```python
from build123d import *

# Parameters (mm, degrees)
SKETCH_6_W           = 28.99281841
SKETCH_6_H           = 28.951324053
EXTRUDE_2_DEPTH      = 10
SKETCH_8_W           = 76
SKETCH_8_H           = 88
EXTRUDE_3_DEPTH      = 4
SKETCH_4_R           = 1.55
CUT_EXTRUDE_2_DEPTH  = 15
SKETCH_5_R           = 1.55
CUT_EXTRUDE_3_DEPTH  = 15
SKETCH_10_W          = 4.022554567
SKETCH_10_H          = 29.702617941
EXTRUDE_9_DEPTH      = 38
SKETCH_11_W          = 4.010171553
SKETCH_11_H          = 29.702617961
EXTRUDE_10_DEPTH     = 38
SKETCH_14_W          = 5
SKETCH_14_H          = 88
EXTRUDE_14_DEPTH     = 50
SKETCH_15_W          = 5
SKETCH_15_H          = 88
EXTRUDE_15_DEPTH     = 50
SKETCH_21_R          = 1.4
CUT_EXTRUDE_8_DEPTH  = 8
CUT_EXTRUDE_9_DEPTH  = 80
CUT_EXTRUDE_11_DEPTH = 80
FILLET_1_R           = 5
FILLET_2_R           = 5
SKETCH_24_W          = 28.984243656
SKETCH_24_H          = 0.299988544
EXTRUDE_16_DEPTH     = 10
SKETCH_25_W          = 37.016969776
SKETCH_25_H          = 2
EXTRUDE_18_DEPTH     = 10
FILLET_7_R           = 2
FILLET_8_R           = 3
FILLET_9_R           = 3
FILLET_10_R          = 3
SKETCH_19_R          = 3.1
CUT_EXTRUDE_12_DEPTH = 3
SKETCH_27_R          = 1.5
CUT_EXTRUDE_13_DEPTH = 10
SKETCH_28_R          = 1.6
CUT_EXTRUDE_15_DEPTH = 15


with BuildPart() as part:
    # 草图6 → 凸台-拉伸2 (new body)
    with BuildSketch(Plane.XZ.offset(14.4)):
        with Locations((0.000972868, 14.775650571)):
            Rectangle(SKETCH_6_W, SKETCH_6_H)
    extrude(amount=EXTRUDE_2_DEPTH)

    # 草图8 → 凸台-拉伸3 (add)
    with BuildSketch(Plane.XZ.offset(24.4)):
        with Locations((1e-09, -13.999999049)):
            Rectangle(SKETCH_8_W, SKETCH_8_H)
    extrude(amount=EXTRUDE_3_DEPTH)

    # 草图4 → 切除-拉伸2 (cut)
    with BuildSketch(Plane.XZ.offset(14.4)):
        with Locations(Location((-10, 2.1, 0), (0, 0, 270))):
            Circle(SKETCH_4_R)
        with Locations(Location((10, 2.1, 0), (0, 0, 270))):
            Circle(SKETCH_4_R)
    extrude(amount=CUT_EXTRUDE_2_DEPTH, mode=Mode.SUBTRACT)

    # 草图5 → 切除-拉伸3 (cut)
    with BuildSketch(Plane.XZ.offset(14.4)):
        with Locations(Location((0, 25.8, 0), (0, 0, 270))):
            Circle(SKETCH_5_R)
    extrude(amount=CUT_EXTRUDE_3_DEPTH, mode=Mode.SUBTRACT)

    # 草图10 → 凸台-拉伸9 (add)
    with BuildSketch(Plane(origin=(0, -24.4, 0), x_dir=(1, 0, 0), z_dir=(0, 1, 0))):
        with Locations((16.503397967, -14.851308971)):
            Rectangle(SKETCH_10_W, SKETCH_10_H)
    extrude(amount=EXTRUDE_9_DEPTH)

    # 草图11 → 凸台-拉伸10 (add)
    with BuildSketch(Plane(origin=(0, -24.4, 0), x_dir=(1, 0, 0), z_dir=(0, 1, 0))):
        with Locations((-16.497208749, -14.851308981)):
            Rectangle(SKETCH_11_W, SKETCH_11_H)
    extrude(amount=EXTRUDE_10_DEPTH)

    # 草图14 → 凸台-拉伸14 (add)
    with BuildSketch(Plane(origin=(0, -24.4, 0), x_dir=(1, 0, 0), z_dir=(0, 1, 0))):
        with Locations((-35.499999999, 13.999999049)):
            Rectangle(SKETCH_14_W, SKETCH_14_H)
    extrude(amount=EXTRUDE_14_DEPTH)

    # 草图15 → 凸台-拉伸15 (add)
    with BuildSketch(Plane(origin=(0, -24.4, 0), x_dir=(1, 0, 0), z_dir=(0, 1, 0))):
        with Locations((35.500000001, 13.999999049)):
            Rectangle(SKETCH_15_W, SKETCH_15_H)
    extrude(amount=EXTRUDE_15_DEPTH)

    # 草图21 → 切除-拉伸8 (cut)
    with BuildSketch(Plane(origin=(0, 25.6, 0), x_dir=(1, 0, 0), z_dir=(0, 1, 0))):
        with Locations(Location((-35.499999999, 52.999999049, 0), (0, 0, 270))):
            Circle(SKETCH_21_R)
        with Locations(Location((-35.499999999, -25.000000951, 0), (0, 0, 270))):
            Circle(SKETCH_21_R)
        with Locations(Location((35.500000001, 52.999999049, 0), (0, 0, 270))):
            Circle(SKETCH_21_R)
        with Locations(Location((35.500000001, -25.000000951, 0), (0, 0, 270))):
            Circle(SKETCH_21_R)
    extrude(amount=-CUT_EXTRUDE_8_DEPTH, mode=Mode.SUBTRACT)

    # 草图22 → 切除-拉伸9 (cut)
    with BuildSketch(Plane.ZY.offset(37.999999999)):
        with BuildLine():
            Line((-37.999999049, 10), (-17.999999049, 10))
            ThreePointArc((-17.999999049, 10), (-7.999999049, 0), (-17.999999049, -10))
            Line((-17.999999049, -10), (-37.999999049, -10))
            ThreePointArc((-37.999999049, -10), (-47.999999049, 0), (-37.999999049, 10))
        make_face()
    extrude(amount=-CUT_EXTRUDE_9_DEPTH, mode=Mode.SUBTRACT)

    # 草图23 → 切除-拉伸11 (cut)
    with BuildSketch(Plane(origin=(0, -24.4, 0), x_dir=(1, 0, 0), z_dir=(0, 1, 0))):
        with BuildLine():
            Line((10, 37.999999049), (10, 17.999999049))
            ThreePointArc((10, 17.999999049), (0, 7.999999049), (-10, 17.999999049))
            Line((-10, 17.999999049), (-10, 37.999999049))
            ThreePointArc((-10, 37.999999049), (0, 47.999999049), (10, 37.999999049))
        make_face()
    extrude(amount=-CUT_EXTRUDE_11_DEPTH, mode=Mode.SUBTRACT)

    # 圆角1
    fillet_1_edges = [part.edges().sort_by_distance(p)[0] for p in [
        (-32.999999999, -24.4, -13.999999049),
    ]]
    fillet(fillet_1_edges, radius=FILLET_1_R)

    # 圆角2
    fillet_2_edges = [part.edges().sort_by_distance(p)[0] for p in [
        (33.000000001, -24.4, -13.999999049),
    ]]
    fillet(fillet_2_edges, radius=FILLET_2_R)

    # 草图24 → 凸台-拉伸16 (add)
    with BuildSketch(Plane(origin=(0, -24.4, 0), x_dir=(1, 0, 0), z_dir=(0, 1, 0))):
        with Locations((-1.144e-06, -0.149994272)):
            Rectangle(SKETCH_24_W, SKETCH_24_H)
    extrude(amount=EXTRUDE_16_DEPTH)

    # 草图25 → 凸台-拉伸18 (add)
    with BuildSketch(Plane(origin=(0, -24.4, 0), x_dir=(1, 0, 0), z_dir=(0, 1, 0))):
        with Locations((0.006190363, 1)):
            Rectangle(SKETCH_25_W, SKETCH_25_H)
    extrude(amount=EXTRUDE_18_DEPTH)

    # 圆角7
    fillet_7_edges = [part.edges().sort_by_distance(p)[0] for p in [
        (0.006190363, -14.4, -2),
    ]]
    fillet(fillet_7_edges, radius=FILLET_7_R)

    # 圆角8
    fillet_8_edges = [part.edges().sort_by_distance(p)[0] for p in [
        (18.514675251, -24.4, 13.85130897),
    ]]
    fillet(fillet_8_edges, radius=FILLET_8_R)

    # 圆角9
    fillet_9_edges = [part.edges().sort_by_distance(p)[0] for p in [
        (1.506190363, -24.4, -2),
    ]]
    fillet(fillet_9_edges, radius=FILLET_9_R)

    # 圆角10
    fillet_10_edges = [part.edges().sort_by_distance(p)[0] for p in [
        (-18.502294525, -24.4, 12.35130898),
    ]]
    fillet(fillet_10_edges, radius=FILLET_10_R)

    # 草图19 → 切除-拉伸12 (cut)
    with BuildSketch(Plane.XZ.offset(28.4)):
        with Locations(Location((0, 25.8, 0), (0, 0, 270))):
            Circle(SKETCH_19_R)
        with Locations(Location((-10, 2.1, 0), (0, 0, 270))):
            Circle(SKETCH_19_R)
        with Locations(Location((10, 2.1, 0), (0, 0, 270))):
            Circle(SKETCH_19_R)
    extrude(amount=-CUT_EXTRUDE_12_DEPTH, mode=Mode.SUBTRACT)

    # 草图27 → 切除-拉伸13 (cut)
    with BuildSketch(Plane(origin=(0, 25.6, 0), x_dir=(1, 0, 0), z_dir=(0, 1, 0))):
        with Locations(Location((35.500000001, 52.999999049, 0), (0, 0, 270))):
            Circle(SKETCH_27_R)
        with Locations(Location((-35.499999999, 52.999999049, 0), (0, 0, 270))):
            Circle(SKETCH_27_R)
        with Locations(Location((-35.499999999, -25.000000951, 0), (0, 0, 270))):
            Circle(SKETCH_27_R)
        with Locations(Location((35.500000001, -25.000000951, 0), (0, 0, 270))):
            Circle(SKETCH_27_R)
    extrude(amount=-CUT_EXTRUDE_13_DEPTH, mode=Mode.SUBTRACT)

    # 草图28 → 切除-拉伸15 (cut)
    with BuildSketch(Plane.XZ.offset(28.4)):
        with Locations(Location((-10, 2.1, 0), (0, 0, 270))):
            Circle(SKETCH_28_R)
        with Locations(Location((10, 2.1, 0), (0, 0, 270))):
            Circle(SKETCH_28_R)
        with Locations(Location((0, 25.8, 0), (0, 0, 270))):
            Circle(SKETCH_28_R)
    extrude(amount=-CUT_EXTRUDE_15_DEPTH, mode=Mode.SUBTRACT)


solid = part.part
```
Input: part model. Units: mm. Frame: model coordinates. A direction names the side the tool comes from. Coordinates: 2 decimals unless noted, no trailing zeros. Loops run counter-clockwise (first coordinate to the right, second up) from the corner with the lowest first, then second, coordinate; pieces in that order, holes last. Notation, with made-up numbers: M 5.5,10 L 39.5,10 A16 ccw 39.5,37 Z; hole C -28.75,-16 d1. An arc over 180 degrees is marked long. Use a Markdown table: item, result. Add a question column.
1) Pin query (flat end, axial travel): P1, Ø5, axis at x = -3.5, z = -42.5, coming from the -Y side; P2, Ø4, axis at x = -10, z = 2.1, coming from the +Y side; P3, Ø6, axis at x = -11.5, y = -13.5, coming from the -Z side; P4, Ø2, axis at x = -17, z = 19.5, coming from the +Y side. Return the tip coordinate at first contact, or that it passes through.
2) Section D-D, the plane z = 2.1. Give the number of separate pieces and of enclosed holes in the cut face, plus the area to 3 significant figures.
3) Set-up query: faces 4 (the flat face through (35, -10, -28)), 5 (the flat face through (16, -6, 29.703)), 6 (the cylindrical face through (0.27, -15, -1.43)), 7 (the flat face through (33, 3, -4)), 8 (the cylindrical face through (0.931, -26.921, 22.843)). Return all of +Z, -Z, +X, -X, +Y, -Y with unobstructed straight access to the full face (end or side cutting, diameter ignored); none if empty.
4) Section C-C, the plane x = 0. Return the cut outline in (y, z).
5) Draft query along Y for faces 1 (the cylindrical face through (35, 0, -48)), 2 (the cylindrical face through (0, -26, -8)), 3 (the cylindrical face through (31.5, -22.97, -14.62)). Return one class per face: +Y half, -Y half, draft (parallel to the pull), parting line (faces both ways), or undercut.
6) Section A-A, the plane x = -35.5. Return the cut outline in (y, z), plus the area to 3 significant figures.
7) Section B-B, the plane z = -19.5. Return the cut outline in (x, y).
8) Line query: L1, parallel to X at y = 12.5, z = 19.5; L2, parallel to X at y = 21.75, z = 25; L3, parallel to X at y = -27.5, z = 2.1. Output: solid intervals per line, ascending. Write a range as from..to.
Answer below:
| question | item | result |
|---|---|---|
| 1 | P1 | through |
| 1 | P2 | y = -14.4 |
| 1 | P3 | z = -2 |
| 1 | P4 | y = 13.6 |
| 2 | separate pieces | 3 |
| 2 | enclosed holes | 0 |
| 2 | area | 1,310 mm2 |
| 3 | face 4 | +X, -X |
| 3 | face 5 | +Z, +Y |
| 3 | face 6 | -Z, +Y |
| 3 | face 7 | +Z, -Z, +Y |
| 3 | face 8 | -Y |
| 4 | outline | M -28.4,-58 L -24.4,-58 L -24.4,-48 L -28.4,-48 Z; M -28.4,-8 L -24.4,-8 L -24.4,-5 A3 cw -21.4,-2 L -16.4,-2 A2 ccw -14.4,0 L -14.4,24.2 L -25.4,24.2 L -25.4,22.7 L -28.4,22.7 Z; M -28.4,28.9 L -25.4,28.9 L -25.4,27.4 L -14.4,27.4 L -14.4,29.25 L -24.4,29.25 L -24.4,30 L -28.4,30 Z |
| 5 | face 1 | undercut |
| 5 | face 2 | draft |
| 5 | face 3 | +Y half |
| 6 | outline | M -28.4,-58 L 25.6,-58 L 25.6,-54.5 L 15.6,-54.5 L 15.6,-51.5 L 25.6,-51.5 L 25.6,23.5 L 15.6,23.5 L 15.6,26.5 L 25.6,26.5 L 25.6,30 L -28.4,30 Z; hole M -10,-38 A10 ccw 10,-38 L 10,-18 A10 ccw -10,-18 Z |
| 6 | area | 3,980 mm2 |
| 7 | outline | M -38,-28.4 L -10,-28.4 L -10,-24.4 L -28,-24.4 A5 cw -33,-19.4 L -33,-10 L -38,-10 Z; M -38,10 L -33,10 L -33,25.6 L -38,25.6 Z; M 10,-28.4 L 38,-28.4 L 38,-10 L 33,-10 L 33,-19.4 A5 cw 28,-24.4 L 10,-24.4 Z; M 33,10 L 38,10 L 38,25.6 L 33,25.6 Z |
| 8 | L1 | -38..-33, -18.5..-14.49, 14.49..18.51, 33..38 |
| 8 | L2 | -38..-37, -34..-33, 33..34, 37..38 |
| 8 | L3 | -38..-13.1, -6.9..6.9, 13.1..38 |
